For this review, use the dimensioned drawing (mm, ordinates from the lowest corner) and the shaded views. Coordinates: 2 decimals unless noted, no trailing zeros. Loops run counter-clockwise (first coordinate to the right, second up) from the corner with the lowest first, then second, coordinate; pieces in that order, holes last. Notation, with made-up numbers: M -3,49.5 L 16,49.5 A28 cw 16,72.5 Z; hole C 73,-34 d11. An arc over 180 degrees is marked long. Write item = value, one per line. Start each with the question number.
Q1. Wall thickness on probe 1 along Z at (x, y) = (239, 11); probe 2 along X at (y, z) = (8.5, 460); probe 3 along Y at (x, z) = (317, 45.5): over which ranges is each line inside the solid? List them lowest first.
Q2. Clearance check with flat-ended pins moving along their axes: pin 1 Ø2 at (x, y) = (405, 3) entering from -Z; pin 2 Ø4 at (y, z) = (15, 658) entering from -X. State where each tip first meets the part, or that it passes through.
Q3. We need section A-A on x = 276. Give the boundary of the cut face in (y, z).
Q4. We need section B-B on z = 181. Give the boundary of the cut face in (x, y).
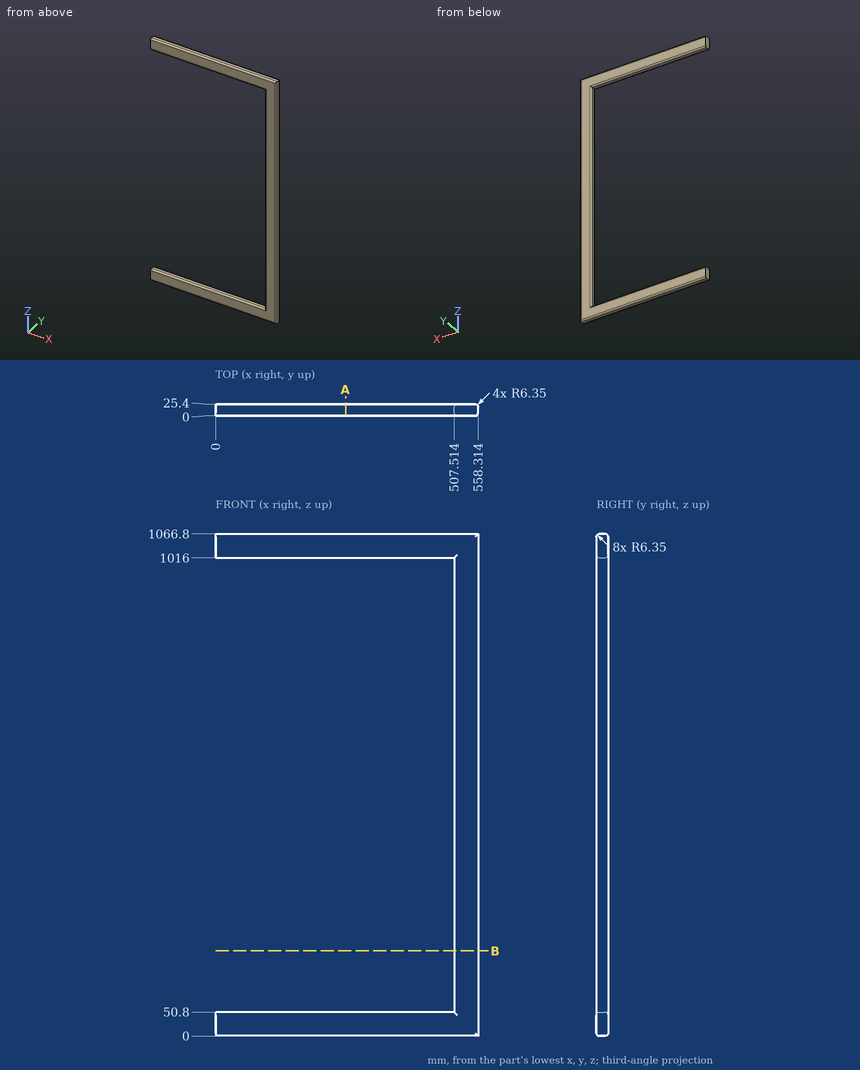
Returned:
q1.probe_1 = 0 to 50.8, 1016 to 1066.8
q1.probe_2 = 507.51 to 558.31
q1.probe_3 = 0.09 to 25.31
q2.pin_1 = 0.45
q2.pin_2 = 507.51
q3.outline = M 0,6.35 A6.35 ccw 6.35,0 L 19.05,0 A6.35 ccw 25.4,6.35 L 25.4,44.45 A6.35 ccw 19.05,50.8 L 6.35,50.8 A6.35 ccw 0,44.45 Z; M 0,1022.35 A6.35 ccw 6.35,1016 L 19.05,1016 A6.35 ccw 25.4,1022.35 L 25.4,1060.45 A6.35 ccw 19.05,1066.8 L 6.35,1066.8 A6.35 ccw 0,1060.45 Z
q4.outline = M 507.51,6.35 A6.35 ccw 513.86,0 L 551.96,0 A6.35 ccw 558.31,6.35 L 558.31,19.05 A6.35 ccw 551.96,25.4 L 513.86,25.4 A6.35 ccw 507.51,19.05 Z
